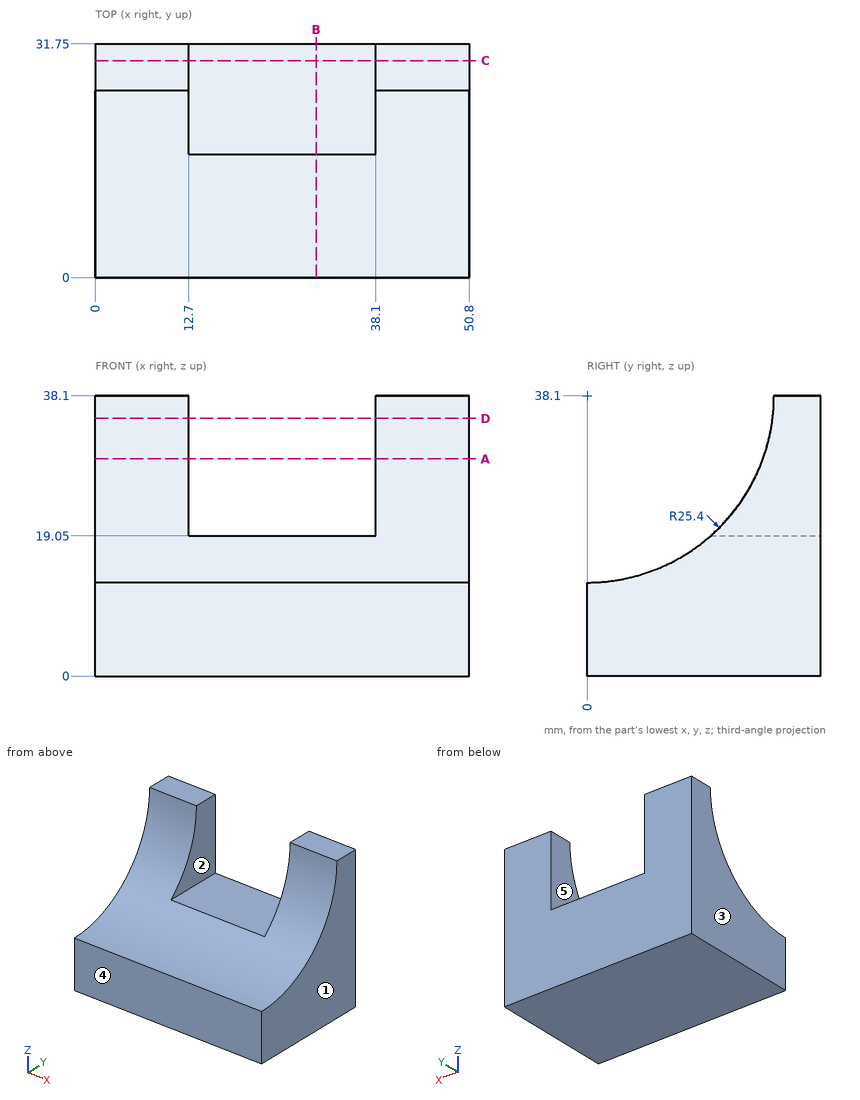
Verification items for this drawing (mm, ordinates from the low corner). A direction names the side the tool comes from. Coordinates: 2 decimals unless noted, no trailing zeros. Order: outer loops, then holes, each group sorted by start corner. A loop starts at its lowest first (then second) coordinate and runs counter-clockwise, first axis right, second up. Notation, with made-up numbers: M -3,68 L 18,68 A17 ccw 18,100 Z; hole C -19.5,-22 d3. An arc over 180 degrees is marked long. One line per item, written item: value. Start each with the question number.
Item 1: Depth check by flat-ended pin: P1, Ø4.5, axis at x = 22, y = 22.5, coming from the +Z side. Enter the tip coordinate at first touch or a pass-through.
Item 2: Sectioned sample at C-C on y = 29.5. Record the cut outline in (x, z).
Item 3: Mould release check, pull along X, two halves, no side actions. Record for the marked faces 1, 2 and 3: pulls with the +X half, pulls with the -X half, needs draft (parallel to the pull), parting line crosses it, or undercut.
Item 4: Sectioned sample at A-A on z = 29.5. Record the cut outline in (x, y), then the cut area to 3 significant figures.
Item 5: Sectioned sample at D-D on z = 35. Record the cut outline in (x, y).
Item 6: Access from +Z, -Z, +X, -X, +Y, -Y to the whole of each face (thin tool, end or side, straight path). Record for the marked faces 4 and 5.
Item 7: Sectioned sample at B-B on x = 30. Record the cut outline in (y, z), then the cut area to 3 significant figures.
Item 8: Thickness scan on probe 1 along X at (y, z) = (26.5, 24.5); probe 2 along Z at (x, y) = (30, 22); probe 3 along Y at (x, z) = (43, 35). Record the ranges inside material, lowest first.
Calculated:
1. P1: z = 19.05
2. outline: M 0,0 L 50.8,0 L 50.8,38.1 L 38.1,38.1 L 38.1,19.05 L 12.7,19.05 L 12.7,38.1 L 0,38.1 Z
3. face 1: pulls with the +X half
3. face 2: undercut
3. face 3: pulls with the -X half
4. outline: M 0,23.9 L 12.7,23.9 L 12.7,31.75 L 0,31.75 Z; M 38.1,23.9 L 50.8,23.9 L 50.8,31.75 L 38.1,31.75 Z
4. area: 199 mm^2
5. outline: M 0,25.21 L 12.7,25.21 L 12.7,31.75 L 0,31.75 Z; M 38.1,25.21 L 50.8,25.21 L 50.8,31.75 L 38.1,31.75 Z
6. face 4: +Z, -Z, +X, -X, -Y
6. face 5: +Z, +Y, -Y
7. outline: M 0,0 L 31.75,0 L 31.75,19.05 L 16.8,19.05 A25.4 cw 0,12.7 Z
7. area: 532 mm^2
8. probe 1: 0 to 12.7, 38.1 to 50.8
8. probe 2: 0 to 19.05
8. probe 3: 25.21 to 31.75
